Can you work these out from the model? Positions are in its coordinate system, mm. A direction names the side the tool comes from. Round coordinates to 2 decimals unless told otherwise and drop trailing zeros. Loops run counter-clockwise (first coordinate to the right, second up) from the corner with the lowest first, then second, coordinate; pieces in that order, holes last. Notation, with made-up numbers: (64.25, 23) - (74.25, 23) arc R17 cw to (74.25, 32) - close; hole circle Ø11 at (87, -36). An arc over 180 degrees is marked (long way). Answer as CSV lines item,"result".
```python
from build123d import *

# Parameters (mm, degrees)
SKETCH_W             = 156
SKETCH_H             = 95
PAD_DEPTH            = 15
SKETCH001_W          = 152
SKETCH001_H          = 91
POCKET_DEPTH         = 8
SKETCH002_W          = 156
SKETCH002_H          = 90
POCKET001_DEPTH      = 5
POCKET001_DEPTH_BACK = -9
SKETCH003_W          = 137.52
SKETCH003_H          = 77.232
POCKET002_DEPTH      = 5
SKETCH004_W          = 15
SKETCH004_H          = 2
PAD001_DEPTH         = 8
SKETCH005_W          = 15
SKETCH005_H          = 2
PAD002_DEPTH         = 8
POCKET003_DEPTH      = 3
POCKET004_DEPTH      = 13
SKETCH008_W          = 12
SKETCH008_H          = 10
POCKET005_DEPTH      = 5


with BuildPart() as part:
    # Sketch → Pad (new body)
    with BuildSketch(Plane.XY):
        Rectangle(SKETCH_W, SKETCH_H)
    extrude(amount=PAD_DEPTH)

    # Sketch001 (on Face6 of Pad) → Pocket (cut)
    with BuildSketch(Plane.XY.offset(15)):
        Rectangle(SKETCH001_W, SKETCH001_H)
    extrude(amount=-POCKET_DEPTH, mode=Mode.SUBTRACT)

    # Sketch002 (on Face11 of Pocket) → Pocket001 (cut, two sides)
    with BuildSketch(Plane.XY.offset(7)) as pocket001_sk:
        Rectangle(SKETCH002_W, SKETCH002_H)
    extrude(amount=-POCKET001_DEPTH, mode=Mode.SUBTRACT)
    extrude(pocket001_sk.sketch, amount=-POCKET001_DEPTH_BACK, mode=Mode.SUBTRACT)

    # Sketch003 (on Face7 of Pocket001) → Pocket002 (cut)
    with BuildSketch(Plane.XY.offset(2)):
        with Locations((1, 3.44)):
            Rectangle(SKETCH003_W, SKETCH003_H)
    extrude(amount=-POCKET002_DEPTH, mode=Mode.SUBTRACT)

    # Sketch004 (on Face16 of Pocket002) → Pad001 (join)
    with BuildSketch(Plane.XZ.offset(-45.5)):
        with Locations((-37.5, 10.5)):
            Rectangle(SKETCH004_W, SKETCH004_H)
        with Locations((37.5, 10.5)):
            Rectangle(SKETCH004_W, SKETCH004_H)
    extrude(amount=PAD001_DEPTH)

    # Sketch005 (on Face22 of Pad001) → Pad002 (join)
    with BuildSketch(Plane(origin=(0, -45.5, 0), x_dir=(-1, 0, 0), z_dir=(0, 1, 0))):
        with Locations((-37.5, 10.5)):
            Rectangle(SKETCH005_W, SKETCH005_H)
    extrude(amount=PAD002_DEPTH)

    # Sketch006 (on Face5 of Pad002) → Pocket003 (cut)
    with BuildSketch(Plane.XY.offset(15)):
        Polygon((-78, -45), (-78, -47.5), (78, -47.5), (78, -45), (76, -45), (76, -45.5), (-76, -45.5), (-76, -45), align=None)
        Polygon((-78, 47.5), (-78, 45), (-76, 45), (-76, 45.5), (76, 45.5), (76, 45), (78, 45), (78, 47.5), align=None)
    extrude(amount=-POCKET003_DEPTH, mode=Mode.SUBTRACT)

    # Sketch007 (on Face4 of Pocket003) → Pocket004 (cut)
    with BuildSketch(Plane.XY.offset(12)):
        with BuildLine():
            Line((-68, -47.5), (-78, -47.5))
            Line((-78, -47.5), (-78, -42.5))
            Line((-78, -42.5), (-70, -42.5))
            ThreePointArc((-68, -44.5), (-68.585786, -43.085786), (-70, -42.5))
            Line((-68, -47.5), (-68, -44.5))
        make_face()
        with BuildLine():
            Line((68, -47.5), (78, -47.5))
            Line((78, -47.5), (78, -42.5))
            Line((78, -42.5), (70, -42.5))
            ThreePointArc((70, -42.5), (68.585786, -43.085786), (68, -44.5))
            Line((68, -47.5), (68, -44.5))
        make_face()
    extrude(amount=-POCKET004_DEPTH, mode=Mode.SUBTRACT)

    # Sketch008 (on Face1 of Pocket004) → Pocket005 (cut)
    with BuildSketch(Plane(origin=(0, 47.5, 0), x_dir=(-1, 0, 0), z_dir=(0, 1, 0))):
        with Locations((-24, 7)):
            Rectangle(SKETCH008_W, SKETCH008_H)
    extrude(amount=-POCKET005_DEPTH, mode=Mode.SUBTRACT)


solid = part.part
```
Q1. Imagine slicing it at D-D (y = -18). Write out the boundary of the cut face in (x, z).
Checks:
outline,"(-78, 0) - (-67.76, 0) - (-67.76, 2) - (-78, 2) - close; (69.76, 0) - (78, 0) - (78, 2) - (69.76, 2) - close"
Q2. If I drill on line 1 along X through (y, z) = (34, 1); line 2 along Y through (x, z) = (61.5, 5.75); line 3 along Y through (x, z) = (0, 8.5), over which ranges is the centre line in solid material (lowest first)? Write a range as [from, to].
Checks:
line 1,"[-78, -67.76], [69.76, 78]"
line 2,"[-47.5, -45], [45, 47.5]"
line 3,"[-47.5, -45.5], [45.5, 47.5]"
Q3. Imagine slicing it at A-A (x = -34). Write out the boundary of the cut face in (y, z).
Checks:
outline,"(-47.5, 0) - (-35.18, 0) - (-35.18, 2) - (-45, 2) - (-45, 7) - (-45.5, 7) - (-45.5, 12) - (-47.5, 12) - close; (37.5, 9.5) - (45.5, 9.5) - (45.5, 7) - (45, 7) - (45, 2) - (42.06, 2) - (42.06, 0) - (47.5, 0) - (47.5, 12) - (45.5, 12) - (45.5, 11.5) - (37.5, 11.5) - close"
Q4. On a 3-axis mill with a long thin cutter (end or side, diameter ignored), from which of +Z, -Z, +X, -X, +Y, -Y can I reach the whole of each face in a straight line? I mean faces 1 (the flat face through (68, -46, 6)), 2 (the flat face through (38, -42, 9.5)), 3 (the flat face through (38, -42, 11.5)), 4 (the flat face through (-1, -47.5, 6)). Say none if no direction works.
Checks:
face 1,"+Z, -Z, +X, -Y"
face 2,"+X, -X"
face 3,"+Z, +X, -X"
face 4,"+Z, -Z, +X, -X, -Y"
Q5. I'm going to push flat-ended pins straight in: pin 1 Ø0.6 at (x, z) = (-72, 1) entering from -Y; pin 2 Ø2 at (y, z) = (42, 11) entering from +X; pin 3 Ø1.5 at (y, z) = (-46.5, 7) entering from -X. Where does each tip first touch, or does it pass through?
Checks:
pin 1,"y = -42.5"
pin 2,"x = 45"
pin 3,"x = -68"
Q6. Imagine slicing it at B-B (y = -39.5). Write out the boundary of the cut face in (x, z), then the cut area to 3 significant figures.
Checks:
outline,"(-78, 0) - (78, 0) - (78, 2) - (-78, 2) - close; (30, 9.5) - (45, 9.5) - (45, 11.5) - (30, 11.5) - close"
area,"342 mm²"
Q7. We'd pull the mould along X, two halves only. Please class faces 5 (the flat face through (30, 45, 10)), 6 (the flat face through (-68, -46, 6)), 7 (the flat face through (-12, -38, 0)), 8 (the flat face through (78, 9, 1)): pulls with the +X half, pulls with the -X half, needs draft (parallel to the pull), parting line crosses it, or undercut.
Checks:
face 5,"undercut"
face 6,"pulls with the -X half"
face 7,"needs draft"
face 8,"pulls with the +X half"
Q8. Imagine slicing it at C-C (x = -64). Write out the boundary of the cut face in (y, z), then the cut area to 3 significant figures.
Checks:
outline,"(-47.5, 0) - (-35.18, 0) - (-35.18, 2) - (-45, 2) - (-45, 7) - (-45.5, 7) - (-45.5, 12) - (-47.5, 12) - close; (42.06, 0) - (47.5, 0) - (47.5, 12) - (45.5, 12) - (45.5, 7) - (45, 7) - (45, 2) - (42.06, 2) - close"
area,"80.5 mm²"
